Answer from the drawing. Dimensions are ordinates in mm from the lowest x, y and z of the part. A direction names the side the tool comes from. Round coordinates to 2 decimals unless told otherwise and drop trailing zeros. Write each loop counter-clockwise with the first axis right and the second up, starting at its lowest first coordinate (ties: lowest second). Pieces come first, ordered by that corner, then holes. Notation, with made-up numbers: M -30,65.5 L 23,65.5 A31 ccw 23,93.5 Z; hole C 44,-3 d6. An arc over 180 degrees is marked long. Answer as CSV lines item,"result". Start each with the question number.
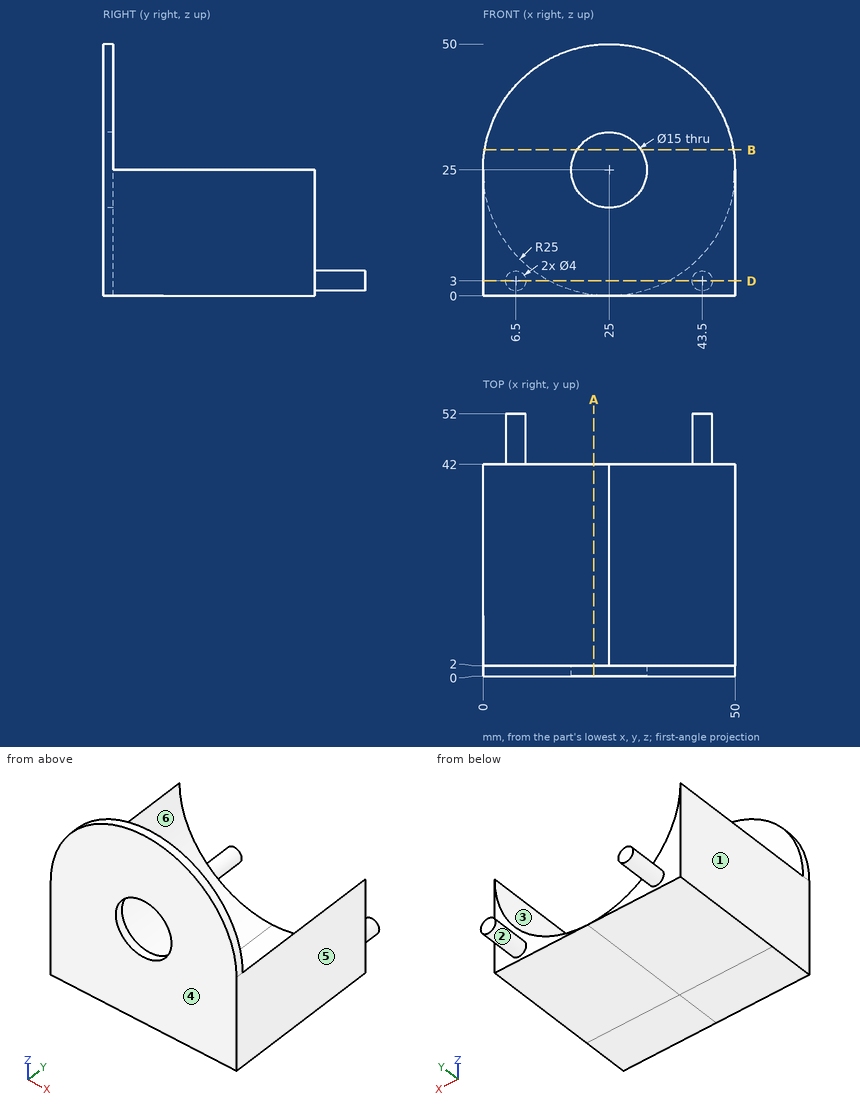
Q1. Find section B-B (z = 29). Determine the outline of the cut face in (x, y), plus the area to 3 significant figures.
Q2. For the marked faces 1, 2 and 3, determine the directions among +Z, -Z, +X, -X, +Y, -Y from which every point of the face is accessible in a straight line to the end or side of a thin tool.
Q3. Straight lines are drawn through the part: L1, parallel to Z at x = 25, y = 1.35; L2, parallel to Z at x = 32, y = 31; L3, parallel to Y at x = 3, z = 21. For each, find the intervals that lie inside material, in ascending order.
Q4. Find section A-A (x = 22). Determine the outline of the cut face in (y, z), plus the area to 3 significant figures.
Q5. Each of these flat-tipped pins is pushed along its axis until it touches: P1, Ø1, axis at x = 29, y = 30.5, coming from the +Z side; P2, Ø3, axis at x = 44, y = 13, coming from the +Z side; P3, Ø1.5, axis at x = 16.5, z = 22.5, coming from the -Y side; P4, Ø8, axis at x = 33.5, y = 21.5, coming from the +Z side. Where does it stop, or does it pass through?
Q6. The mould has two halves that part along X. Classify the marked faces 4, 5 and 6: +X half, -X half, draft (parallel to the pull), parting line (faces both ways), or undercut.
Q7. Find section D-D (z = 3). Determine the outline of the cut face in (x, y).
Reported:
1,outline,"M 0.32,0 L 18.66,0 L 18.66,2 L 0.32,2 Z; M 31.34,0 L 49.68,0 L 49.68,2 L 31.34,2 Z"
1,area,"73.3 mm2"
2,face 1,"+Z, -Z, -X, +Y, -Y"
2,face 2,"+Y"
2,face 3,"+Z, +Y"
3,L1,"z = 0 to 17.5, 32.5 to 50"
3,L2,"z = 0 to 1"
3,L3,"y = 0 to 2"
4,outline,"M 0,0 L 42,0 L 42,0.18 L 2,0.18 L 2,18.13 L 0,18.13 Z; M 0,31.87 L 2,31.87 L 2,49.82 L 0,49.82 Z"
4,area,"79.4 mm2"
5,P1,"stops at z = 0.41"
5,P2,"stops at z = 10.69"
5,P3,"stops at y = 0"
5,P4,"stops at z = 3.35"
6,face 4,"draft"
6,face 5,"+X half"
6,face 6,"undercut"
7,outline,"M 0,0 L 50,0 L 50,42 L 45.5,42 L 45.5,52 L 41.5,52 L 41.5,42 L 36.87,42 L 36.87,2 L 13.13,2 L 13.13,42 L 8.5,42 L 8.5,52 L 4.5,52 L 4.5,42 L 0,42 Z"
